from build123d import *

# Parameters (mm, degrees)
F1_DEPTH      = 30
F3_DEPTH      = 25
F3_DEPTH_BACK = 40
F5_W          = 20
F5_H          = 30
F6_DEPTH      = 90
F7_R          = 5
F9_DEPTH      = 25
F9_DEPTH_BACK = 40


with BuildPart() as f1:
    # F0 (on Front) → F1 (new body)
    with BuildSketch(Plane.XZ):
        with BuildLine():
            Line((10, -45), (-10, -45))
            Line((-10, -45), (-25, -45))
            ThreePointArc((-25, -45), (-32.071068, -47.928932), (-35, -55))
            Line((-35, -55), (-35, -95))
            ThreePointArc((-35, -95), (-32.071068, -102.071068), (-25, -105))
            Line((-25, -105), (25, -105))
            ThreePointArc((25, -105), (32.071068, -102.071068), (35, -95))
            Line((35, -95), (35, -55))
            ThreePointArc((35, -55), (32.071068, -47.928932), (25, -45))
            Line((25, -45), (10, -45))
        make_face()
    extrude(amount=F1_DEPTH)


with BuildPart() as f3:
    # F2 (on face) → F3 (new body, two sides)
    with BuildSketch(Plane.XZ.offset(30)) as f3_sk:
        Polygon((25, -55), (-25, -55), (-25, -65), (-15, -65), (-15, -85), (-25, -85), (-25, -95), (25, -95), (25, -85), (15, -85), (15, -65), (25, -65), align=None)
    extrude(amount=F3_DEPTH)
    extrude(f3_sk.sketch, amount=-F3_DEPTH_BACK)


with BuildPart() as f1_1:
    add(f1.part)

    # F4: cut F3
    add(f3.part, mode=Mode.SUBTRACT)

    # F5 (on face) → F6 (join)
    with BuildSketch(Plane.XY.offset(-45)):
        with Locations((0, -15)):
            Rectangle(F5_W, F5_H)
    extrude(amount=F6_DEPTH)

    # F7
    f7_edges = [f1_1.edges().sort_by_distance(p)[0] for p in [
        (0, -30, 45),
        (0, 0, 45),
    ]]
    fillet(f7_edges, radius=F7_R)


with BuildPart() as f9:
    # F8 (on face) → F9 (new body, two sides)
    with BuildSketch(Plane.YZ.offset(10)) as f9_sk:
        with BuildLine():
            Line((-10, -35), (-10, 35))
            ThreePointArc((-10, 35), (-15, 40), (-20, 35))
            Line((-20, 35), (-20, -35))
            ThreePointArc((-20, -35), (-15, -40), (-10, -35))
        make_face()
    extrude(amount=F9_DEPTH)
    extrude(f9_sk.sketch, amount=-F9_DEPTH_BACK)


with BuildPart() as f1_2:
    add(f1_1.part)

    # F10: cut F9
    add(f9.part, mode=Mode.SUBTRACT)


solid = f1_2.part
Verification items for the finished model (mm, model axes). A direction names the side the tool comes from. Give positions to 0.01 mm unless a question says otherwise; leave off trailing zeros. Order: outer loops, then holes, each group sorted by start corner. A loop starts at its lowest first (then second) coordinate and runs counter-clockwise, first axis right, second up. Notation, with made-up numbers: (87, -22.5) -> (104, -22.5) arc R9 ccw to (104, -18.5) -> close; hole circle Ø3 at (-7, -35). An arc over 180 degrees is marked (long way). Answer as CSV lines item,"result".
Q1. Depth check by flat-ended pin: pin 1 (10 mm diameter, centred on y = -22.5, z = -11.5, fed in from -X); pin 2 (8 mm diameter, centred on y = -13.5, z = -26.5, fed in from +X); pin 3 (4 mm diameter, centred on x = -10.5, y = -17, fed in from +Z); pin 4 (7.5 mm diameter, centred on x = 20.5, y = -14, fed in from +Z). Enter the tip coordinate at first touch or a pass-through.
Solutions:
pin 1,"stops at x = -10"
pin 2,"stops at x = 10"
pin 3,"stops at z = 45"
pin 4,"stops at z = -45"
Q2. Access from +Z, -Z, +X, -X, +Y, -Y to the whole of each face (thin tool, end or side, straight path). Record for faces 1 (the flat face through (-20, -15, -65)), 2 (the cylindrical face through (0, -15, 40)), 3 (the flat face through (-10, -9, -1)), 4 (the flat face through (35, -15, -75)), 5 (the flat face through (10, -9, -1)).
Solutions:
face 1,"+Y, -Y"
face 2,"+X, -X"
face 3,"+Z, -X, +Y, -Y"
face 4,"+Z, -Z, +X, +Y, -Y"
face 5,"+Z, +X, +Y, -Y"
Q3. Sectioned sample at D-D on z = -26. Record the cut outline in (x, y), plus the area to 3 significant figures.
Solutions:
outline,"(-10, -30) -> (10, -30) -> (10, -20) -> (-10, -20) -> close; (-10, -10) -> (10, -10) -> (10, 0) -> (-10, 0) -> close"
area,"400 mm²"
Q4. Sectioned sample at B-B on y = -15. Record the cut outline in (x, z).
Solutions:
outline,"(-35, -95) arc R10 ccw to (-25, -105) -> (25, -105) arc R10 ccw to (35, -95) -> (35, -55) arc R10 ccw to (25, -45) -> (10, -45) -> (10, -40) -> (-10, -40) -> (-10, -45) -> (-25, -45) arc R10 ccw to (-35, -55) -> close; (-10, 40) -> (10, 40) -> (10, 45) -> (-10, 45) -> close; hole (-25, -95) -> (25, -95) -> (25, -85) -> (15, -85) -> (15, -65) -> (25, -65) -> (25, -55) -> (-25, -55) -> (-25, -65) -> (-15, -65) -> (-15, -85) -> (-25, -85) -> close"
Q5. Scan lines: probe 1 along Z at (x, y) = (-2, -15); probe 2 along Z at (x, y) = (20, -18); probe 3 along X at (y, z) = (-4.25, -92.5). Record each from-to range of solid material in increasing order.
Solutions:
probe 1,"z = -105 to -95, -55 to -40, 40 to 45"
probe 2,"z = -105 to -95, -85 to -65, -55 to -45"
probe 3,"x = -35 to -25, 25 to 35"
Q6. Release check for a two-part mould opening along X. For faces 6 (the flat face through (18, -15, -45)), 7 (the cylindrical face through (-32.15, -14.79, -101.99)), 8 (the flat face through (20, -15, -65)), 9 (the flat face through (0, -15, -95)) record: +X half, -X half, draft (parallel to the pull), parting line (faces both ways), or undercut.
Solutions:
face 6,"draft"
face 7,"-X half"
face 8,"undercut"
face 9,"undercut"
Q7. Sectioned sample at C-C on x = 19. Record the cut outline in (y, z).
Solutions:
outline,"(-30, -105) -> (0, -105) -> (0, -95) -> (-30, -95) -> close; (-30, -85) -> (0, -85) -> (0, -65) -> (-30, -65) -> close; (-30, -55) -> (0, -55) -> (0, -45) -> (-30, -45) -> close"
Q8. Sectioned sample at A-A on x = -1.5. Record the cut outline in (y, z).
Solutions:
outline,"(-30, -105) -> (0, -105) -> (0, -95) -> (-30, -95) -> close; (-30, -55) -> (0, -55) -> (0, 40) arc R5 ccw to (-5, 45) -> (-25, 45) arc R5 ccw to (-30, 40) -> close; hole (-20, -35) arc R5 ccw to (-10, -35) -> (-10, 35) arc R5 ccw to (-20, 35) -> close"
